```python
from build123d import *

# Parameters (mm, degrees)
SKETCH_1_R          = 1
EXTRUDE_2_DEPTH     = 2
SKETCH_3_R          = 1
CUT_EXTRUDE_1_DEPTH = 2
SKETCH_4_R          = 1
EXTRUDE_4_DEPTH     = 2
SKETCH_5_R          = 3
SKETCH_5_R_2        = 1.25
CUT_EXTRUDE_2_DEPTH = 2
EXTRUDE_START       = -2
SKETCH_6_R          = 1
EXTRUDE_6_DEPTH     = 2
SKETCH_7_R          = 1
CUT_EXTRUDE_3_DEPTH = 2
FILLET_3_R          = 1
FILLET_4_R          = 1
FILLET_5_R          = 1


with BuildPart() as part:
    # 草圖1 → 填料-伸長2 (new body)
    with BuildSketch(Plane.XY):
        with BuildLine():
            Line((21.259390326, 6.277522936), (21.259390326, 4.277522936))
            ThreePointArc((21.259390326, 4.277522936), (20.259390326, 3.277522936), (21.259390326, 2.277522936))
            Line((21.259390326, 2.277522936), (23.259390326, 2.277522936))
            Line((23.259390326, 2.277522936), (23.259390326, -1.722477064))
            Line((23.259390326, -1.722477064), (21.259390326, -1.722477064))
            ThreePointArc((21.259390326, -1.722477064), (20.259390326, -2.722477064), (21.259390326, -3.722477064))
            Line((21.259390326, -3.722477064), (21.259390326, -7.722477064))
            ThreePointArc((21.259390326, -7.722477064), (20.259390326, -8.722477064), (21.259390326, -9.722477064))
            Line((21.259390326, -9.722477064), (23.259390326, -9.722477064))
            Line((23.259390326, -9.722477064), (23.259390326, -13.722477064))
            Line((23.259390326, -13.722477064), (21.259390326, -13.722477064))
            ThreePointArc((21.259390326, -13.722477064), (20.259390326, -14.722477064), (21.259390326, -15.722477064))
            Line((21.259390326, -15.722477064), (21.259390326, -17.722477064))
            Line((21.259390326, -17.722477064), (-26.340609674, -17.722477064))
            Line((-26.340609674, -17.722477064), (-26.340609674, -15.722477064))
            ThreePointArc((-26.340609674, -15.722477064), (-25.340609674, -14.722477064), (-26.340609674, -13.722477064))
            Line((-26.340609674, -13.722477064), (-28.340609674, -13.722477064))
            Line((-28.340609674, -13.722477064), (-28.340609674, -9.722477064))
            Line((-28.340609674, -9.722477064), (-26.340609674, -9.722477064))
            ThreePointArc((-26.340609674, -9.722477064), (-25.340609674, -8.722477064), (-26.340609674, -7.722477064))
            Line((-26.340609674, -7.722477064), (-26.340609674, -3.722477064))
            ThreePointArc((-26.340609674, -3.722477064), (-25.340609674, -2.722477064), (-26.340609674, -1.722477064))
            Line((-26.340609674, -1.722477064), (-28.340609674, -1.722477064))
            Line((-28.340609674, -1.722477064), (-28.340609674, 2.277522936))
            Line((-28.340609674, 2.277522936), (-26.340609674, 2.277522936))
            ThreePointArc((-26.340609674, 2.277522936), (-25.340609674, 3.277522936), (-26.340609674, 4.277522936))
            Line((-26.340609674, 4.277522936), (-26.340609674, 6.277522936))
            Line((-26.340609674, 6.277522936), (21.259390326, 6.277522936))
        make_face()
        with Locations((-20.540609674, -5.722477064)):
            Circle(SKETCH_1_R, mode=Mode.SUBTRACT)
        with Locations(Location((15.459390326, -5.722477064, 0), (0, 0, 180))):
            Circle(SKETCH_1_R, mode=Mode.SUBTRACT)
    extrude(amount=EXTRUDE_2_DEPTH)

    # 草圖3 → 除料-伸長1 (cut)
    with BuildSketch(Plane.XY.offset(2)):
        with Locations((19.259390326, -5.722477064)):
            Circle(SKETCH_3_R)
        with Locations(Location((-24.340609674, -3.722477064, 0), (0, 0, 180))):
            Circle(SKETCH_3_R)
    extrude(amount=-CUT_EXTRUDE_1_DEPTH, mode=Mode.SUBTRACT)

    # 草圖4 → 填料-伸長4 (add)
    with BuildSketch(Plane(origin=(0, 0, 0), x_dir=(-1, 0, 0), z_dir=(0, 0, -1))):
        with Locations((-15.459390326, -5.722477064)):
            Circle(SKETCH_4_R)
        with Locations((20.540609674, -5.722477064)):
            Circle(SKETCH_4_R)
    extrude(amount=-EXTRUDE_4_DEPTH)

    # 草圖5 → 除料-伸長2 (cut)
    with BuildSketch(Plane(origin=(0, 0, 0), x_dir=(-1, 0, 0), z_dir=(0, 0, -1))):
        with Locations((2.540609674, -5.722477064)):
            Circle(SKETCH_5_R)
        with Locations((2.540609674, 1.277522936)):
            Circle(SKETCH_5_R_2)
        with Locations((7.490357142, -0.772729596)):
            Circle(SKETCH_5_R_2)
        with Locations((9.540609674, -5.722477064)):
            Circle(SKETCH_5_R_2)
        with Locations((7.490357142, -10.672224533)):
            Circle(SKETCH_5_R_2)
        with Locations((2.540609674, -12.722477064)):
            Circle(SKETCH_5_R_2)
        with Locations((-2.409137794, -10.672224533)):
            Circle(SKETCH_5_R_2)
        with Locations((-4.459390326, -5.722477064)):
            Circle(SKETCH_5_R_2)
        with Locations((-2.409137794, -0.772729596)):
            Circle(SKETCH_5_R_2)
    extrude(amount=-CUT_EXTRUDE_2_DEPTH, mode=Mode.SUBTRACT)

    # 草圖6 → 填料-伸長6 (add)
    with BuildSketch(Plane(origin=(0, 0, 0), x_dir=(-1, 0, 0), z_dir=(0, 0, -1)).offset(EXTRUDE_START)):
        with Locations((-19.259390326, -5.722477064)):
            Circle(SKETCH_6_R)
        with Locations((24.340609674, -3.722477064)):
            Circle(SKETCH_6_R)
    extrude(amount=EXTRUDE_6_DEPTH)

    # 草圖7 → 除料-伸長3 (cut)
    with BuildSketch(Plane(origin=(0, 0, 0), x_dir=(-1, 0, 0), z_dir=(0, 0, -1))):
        with Locations((-19.259390326, 0.277522936)):
            Circle(SKETCH_7_R)
        with Locations((-19.259390326, -11.722477064)):
            Circle(SKETCH_7_R)
        with Locations((24.340609674, -11.722477064)):
            Circle(SKETCH_7_R)
        with Locations((24.340609674, 0.277522936)):
            Circle(SKETCH_7_R)
    extrude(amount=-CUT_EXTRUDE_3_DEPTH, mode=Mode.SUBTRACT)

    # 圓角3
    fillet_3_edges = [part.edges().sort_by_distance(p)[0] for p in [
        (21.259390326, 6.277522936, 1),
    ]]
    fillet(fillet_3_edges, radius=FILLET_3_R)

    # 圓角4
    fillet_4_edges = [part.edges().sort_by_distance(p)[0] for p in [
        (21.259390326, -17.722477064, 1),
    ]]
    fillet(fillet_4_edges, radius=FILLET_4_R)

    # 圓角5
    fillet_5_edges = [part.edges().sort_by_distance(p)[0] for p in [
        (-26.340609674, 6.277522936, 1),
        (-26.340609674, -17.722477064, 1),
    ]]
    fillet(fillet_5_edges, radius=FILLET_5_R)


solid = part.part
```
Can you work these out from the model? Positions are in its coordinate system, mm. A direction names the side the tool comes from. Round coordinates to 2 decimals unless told otherwise and drop trailing zeros. Loops run counter-clockwise (first coordinate to the right, second up) from the corner with the lowest first, then second, coordinate; pieces in that order, holes last. Notation, with made-up numbers: (-33.75, 82.5) -> (-2.75, 82.5) arc R10 cw to (-2.75, 90.5) -> close; hole circle Ø7 at (-27, 14). An arc over 180 degrees is marked (long way). One line per item, written item: value. Start each with the question number.
1. If I drill on probe 1 along X at (y, z) = (-5.75, 1.2); probe 2 along Y at (x, z) = (2.5, 0.15); probe 3 along Y at (x, z) = (-7, 1), over which ranges is the centre line in solid material (lowest first)?
2. If we mould it in two halves opening along X, with no side actions, what happens to faces 1 (the cylindrical face through (-8.683, -0.397, 0.986)), 2 (the cylindrical face through (-26.04, 5.99, 1.01)), 3 (the flat face through (-8, -6, 0))? For each: pulls with the +X half, pulls with the -X half, needs draft (parallel to the pull), parting line crosses it, or undercut.
3. If we section it at A-A, the plane x = 0: Write out the boundary of the cut face in (y, z), then the cut area to 3 significant figures.
4. For faces 4 (the flat face through (-3, 6.278, 1)), 5 (the flat face through (-27, -9.722, 1)), 6 (the flat face through (21.259, -6, 1)), 7 (the flat face through (-26.341, 5, 1)), which set-ups out of +Z, -Z, +X, -X, +Y, -Y let a thin tool reach every point of the face, with its end or its side?
5. For pin 1 (0.6 mm diameter, centred on x = 22, z = 1, fed in from +Y); pin 2 (0.6 mm diameter, centred on y = -5.5, z = 0.5, fed in from +X), each with a flat end and sliding along its axis, tell me the tip position at first contact or that it passes through.
6. If we section it at C-C, the plane z = 1.5: Give the number of separate pieces and of enclosed holes in the cut face, then the cut area to 3 significant figures.
7. If we section it at B-B, the plane y = -6.5: Write out the boundary of the cut face in (x, z).
Calculated:
1. probe 1: x = -26.34 to -10.79, -8.29 to -5.54, 0.46 to 3.21, 5.71 to 21.26
1. probe 2: y = -17.72 to -11.92, -9.43 to -2.02, 0.47 to 6.28
1. probe 3: y = -17.72 to -11.82, -9.52 to -1.92, 0.38 to 6.28
2. face 1: undercut
2. face 2: pulls with the -X half
2. face 3: needs draft
3. outline: (-17.72, 0) -> (-7.32, 0) -> (-7.32, 2) -> (-17.72, 2) -> close; (-4.13, 0) -> (6.28, 0) -> (6.28, 2) -> (-4.13, 2) -> close
3. area: 41.6 mm²
4. face 4: +Z, -Z, +X, -X, +Y
4. face 5: +Z, -Z, -X
4. face 6: +Z, -Z, +X
4. face 7: +Z, -Z, -X, +Y
5. pin 1: stops at y = 2.28
5. pin 2: stops at x = 21.26
6. separate pieces: 1
6. enclosed holes: 13
6. area: 1,080 mm²
7. outline: (-26.34, 0) -> (-10.52, 0) -> (-10.52, 2) -> (-26.34, 2) -> close; (-8.56, 0) -> (-5.44, 0) -> (-5.44, 2) -> (-8.56, 2) -> close; (0.36, 0) -> (3.48, 0) -> (3.48, 2) -> (0.36, 2) -> close; (5.44, 0) -> (21.26, 0) -> (21.26, 2) -> (5.44, 2) -> close
